Geometry: final body of the model. Coordinates: model frame, mm. A direction names the side the tool comes from. Coordinates: 2 decimals unless noted, no trailing zeros. Order: outer loops, then holes, each group sorted by start corner. A loop starts at its lowest first (then second) coordinate and runs counter-clockwise, first axis right, second up. Notation, with made-up numbers: M 57,-11 L 71,-11 A14 cw 71,5 Z; hole C -12.5,29 d4. An arc over 180 degrees is marked long. Use CSV: the item, a comma, the result in double quotes. Start each with the question number.
Q1. Section query C-C, the plane x = 6. State how many separate pieces and enclosed holes the cut face has, and give its area (3 significant figures).
Q2. Mould query, pull axis Y, two halves, no side actions, for faces 3 (the face through (28.385, -25.229, 1.014)), 4 (the face through (31.48, -1, 1)), 5 (the face through (28.385, -0.479, 1.014)), 6 (the face through (-30.767, 53.248, 1.014)). Classes: +Y half, -Y half, draft (parallel to the pull), parting line (faces both ways), or undercut.
Q3. Section query B-B, the plane y = 49.5. Output: boundary loops of the cut face in (x, z).
Q4. First-contact query: P1, Ø4, axis at x = -27.23, y = 0, coming from the -Z side. Flat tip, straight axial feed; report the tip coordinate or a pass-through.
Q5. Access query for faces 1 (the face through (0, 1, 0)), 2 (the face through (-7, 40.5, 1)). Directions: +Z, -Z, +X, -X, +Y, -Y. A direction counts if a zero-diameter tool reaches every point of the face in a straight line with its end or side. Return the directions, or none.
Q6. Ray query, probe 1 along Y at (x, z) = (-27.23, 1.2); probe 2 along X at (y, z) = (-17.5, 0.55); probe 3 along X at (y, z) = (38.5, 1.9). Return the intervals inside material, ascending.
Q7. Section query A-A, the plane x = -27.23. Output: boundary loops of the cut face in (y, z).
from build123d import *

# Parameters (mm, degrees)
SKETCH1_W           = 62.96
SKETCH1_H           = 108
BOSS_EXTRUDE1_DEPTH = 2
FILLET1_R           = 2.5
SKETCH2_R           = 1.25
CUT_EXTRUDE1_DEPTH  = 2
SKETCH3_R           = 2.5
SKETCH3_R_2         = 2
SKETCH3_W           = 32.96
SKETCH3_H           = 1.138869598
CUT_EXTRUDE2_DEPTH  = 2


with BuildPart() as part:
    # Sketch1 → Boss-Extrude1 (new body)
    with BuildSketch(Plane.XY):
        Rectangle(SKETCH1_W, SKETCH1_H)
    extrude(amount=BOSS_EXTRUDE1_DEPTH)

    # Fillet1
    fillet1_edges = [part.edges().sort_by_distance(p)[0] for p in [
        (31.48, -54, 1),
        (-31.48, -54, 1),
        (-31.48, 54, 1),
        (31.48, 54, 1),
    ]]
    fillet(fillet1_edges, radius=FILLET1_R)

    # Sketch2 → Cut-Extrude1 (cut)
    with BuildSketch(Plane.XY.offset(2)):
        with Locations((-27.23, 49.5)):
            Circle(SKETCH2_R)
        with Locations((27.23, 49.5)):
            Circle(SKETCH2_R)
        with Locations((27.23, 24.75)):
            Circle(SKETCH2_R)
        with Locations((27.23, 0)):
            Circle(SKETCH2_R)
        with Locations((27.23, -24.75)):
            Circle(SKETCH2_R)
        with Locations((27.23, -49.5)):
            Circle(SKETCH2_R)
        with Locations((-27.23, 24.75)):
            Circle(SKETCH2_R)
        with Locations((-27.23, 0)):
            Circle(SKETCH2_R)
        with Locations((-27.23, -24.75)):
            Circle(SKETCH2_R)
        with Locations((-27.23, -49.5)):
            Circle(SKETCH2_R)
    extrude(amount=-CUT_EXTRUDE1_DEPTH, mode=Mode.SUBTRACT)

    # Sketch3 → Cut-Extrude2 (cut)
    with BuildSketch(Plane.XY.offset(2)):
        with Locations((16.48, 39)):
            Circle(SKETCH3_R)
        with Locations((-16.48, 39)):
            Circle(SKETCH3_R_2)
        with BuildLine():
            Line((-9.48, 40.5), (-3.48, 40.5))
            ThreePointArc((-3.48, 40.5), (-1.98, 39), (-3.48, 37.5))
            Line((-3.48, 37.5), (-9.48, 37.5))
            ThreePointArc((-9.48, 37.5), (-10.98, 39), (-9.48, 40.5))
        make_face()
        with Locations((0, -12.5)):
            Rectangle(SKETCH3_W, SKETCH3_H)
        with Locations((0, -10)):
            Rectangle(SKETCH3_W, SKETCH3_H)
        with Locations((0, -15)):
            Rectangle(SKETCH3_W, SKETCH3_H)
        with Locations((0, -17.5)):
            Rectangle(SKETCH3_W, SKETCH3_H)
        with Locations((0, -20)):
            Rectangle(SKETCH3_W, SKETCH3_H)
        with Locations((0, -22.5)):
            Rectangle(SKETCH3_W, SKETCH3_H)
        with Locations((0, -25)):
            Rectangle(SKETCH3_W, SKETCH3_H)
        with Locations((0, -27.5)):
            Rectangle(SKETCH3_W, SKETCH3_H)
        with Locations((0, -30)):
            Rectangle(SKETCH3_W, SKETCH3_H)
        with Locations((0, -32.5)):
            Rectangle(SKETCH3_W, SKETCH3_H)
    extrude(amount=-CUT_EXTRUDE2_DEPTH, mode=Mode.SUBTRACT)


solid = part.part
Responses:
1,separate pieces,"11"
1,enclosed holes,"0"
1,area,"193 mm²"
2,face 3,"undercut"
2,face 4,"draft"
2,face 5,"undercut"
2,face 6,"+Y half"
3,outline,"M -31.48,0 L -28.48,0 L -28.48,2 L -31.48,2 Z; M -25.98,0 L 25.98,0 L 25.98,2 L -25.98,2 Z; M 28.48,0 L 31.48,0 L 31.48,2 L 28.48,2 Z"
4,P1,"stops at z = 0"
5,face 1,"-Z, +X, -X, +Y, -Y"
5,face 2,"+Z, -Z"
6,probe 1,"y = -54 to -50.75, -48.25 to -26, -23.5 to -1.25, 1.25 to 23.5, 26 to 48.25, 50.75 to 54"
6,probe 2,"x = -31.48 to -16.48, 16.48 to 31.48"
6,probe 3,"x = -31.48 to -18.42, -14.54 to -10.89, -2.07 to 14.03, 18.93 to 31.48"
7,outline,"M -54,0 L -50.75,0 L -50.75,2 L -54,2 Z; M -48.25,0 L -26,0 L -26,2 L -48.25,2 Z; M -23.5,0 L -1.25,0 L -1.25,2 L -23.5,2 Z; M 1.25,0 L 23.5,0 L 23.5,2 L 1.25,2 Z; M 26,0 L 48.25,0 L 48.25,2 L 26,2 Z; M 50.75,0 L 54,0 L 54,2 L 50.75,2 Z"
